from build123d import *

# Parameters (mm, degrees)
SKETCH1_R           = 46.5455
SKETCH1_R_2         = 2.60858
BOSS_EXTRUDE1_DEPTH = 3.1242
SKETCH1_5_R         = 47.498
SKETCH1_5_R_2       = 46.5455
BOSS_EXTRUDE2_DEPTH = 8.636
FILLET1_R           = 1.27
FILLET2_R           = 1.27
SKETCH2_R           = 46.4312
BOSS_EXTRUDE3_DEPTH = 0.508
SKETCH3_R           = 46.4312
BOSS_EXTRUDE4_DEPTH = 0.762


with BuildPart() as part:
    # Sketch1 → Boss-Extrude1 (new body)
    # profile 1 of 3: a face of its own
    with BuildSketch(Plane(origin=(0, 0, 0), x_dir=(1, 0, 0), z_dir=(0, 1, 0))):
        with Locations(Location((0, 0, 0), (0, 0, 270))):
            Circle(SKETCH1_R)
        Circle(SKETCH1_R_2, mode=Mode.SUBTRACT)
    # profile 2 of 3: a face of its own
    with BuildSketch(Plane(origin=(0, 0, 0), x_dir=(1, 0, 0), z_dir=(0, 1, 0))):
        with BuildLine():
            ThreePointArc((2.60858, 0), (2.193727268, 1.411470966), (1.081120394, 2.37399838))
            Line((1.081120394, 2.37399838), (2.175329976, -1.439662846))
            ThreePointArc((2.175329976, -1.439662846), (2.497920324, -0.751720475), (2.60858, 0))
        make_face()
    # profile 3 of 3: a face of its own
    with BuildSketch(Plane(origin=(0, 0, 0), x_dir=(1, 0, 0), z_dir=(0, 1, 0))):
        with BuildLine():
            Line((-1.081120394, -2.37399838), (-2.175329976, 1.439662846))
            ThreePointArc((-2.175329976, 1.439662846), (-2.507413058, -0.719422946), (-1.081120394, -2.37399838))
        make_face()
    extrude(amount=BOSS_EXTRUDE1_DEPTH)

    # Sketch1<5> → Boss-Extrude2 (add)
    with BuildSketch(Plane(origin=(0, 0, 0), x_dir=(1, 0, 0), z_dir=(0, 1, 0))):
        with Locations(Location((0, 0, 0), (0, 0, 270))):
            Circle(SKETCH1_5_R)
        with Locations(Location((0, 0, 0), (0, 0, 270))):
            Circle(SKETCH1_5_R_2, mode=Mode.SUBTRACT)
    extrude(amount=BOSS_EXTRUDE2_DEPTH)

    # Fillet1
    fillet1_edges = [part.edges().sort_by_distance(p)[0] for p in [
        (0, 0, -47.498),
    ]]
    fillet(fillet1_edges, radius=FILLET1_R)

    # Fillet2
    # the kernel refuses this fillet: 1.27 mm, written as the material it takes off along each edge
    with BuildSketch(Plane(origin=(0, 8.636, 0), x_dir=(0, 0, 1), z_dir=(-1, 0, 0))) as fillet2_piece_1:
        with BuildLine():
            CenterArc((46.228, -1.229672212), FILLET2_R, 0, 75.522487814)
            Line((46.5455, 0), (46.55185, 0.024593444))
            ThreePointArc((46.55185, 0.024593444), (47.02175, 0.0254), (47.498, 0.0254))
            Line((47.498, 0.0254), (47.5234, 0))
            Line((47.5234, 0), (47.5234, -1.229672212))
            Line((47.5234, -1.229672212), (47.498, -1.229672212))
        make_face()
    revolve(axis=Axis((0, 8.636, 0), (0, 1, 0)), mode=Mode.SUBTRACT)

    # Sketch2 → Boss-Extrude3 (add)
    with BuildSketch(Plane(origin=(0, 3.1242, 0), x_dir=(1, 0, 0), z_dir=(0, 1, 0))):
        with Locations(Location((0, 0, 0), (0, 0, 270))):
            Circle(SKETCH2_R)
        with BuildLine():
            Line((-1.081120394, -2.37399838), (-2.175329976, 1.439662846))
            ThreePointArc((-2.175329976, 1.439662846), (-0.719422946, 2.507413058), (1.081120394, 2.37399838))
            Line((1.081120394, 2.37399838), (2.175329976, -1.439662846))
            ThreePointArc((2.175329976, -1.439662846), (0.719422946, -2.507413058), (-1.081120394, -2.37399838))
        make_face(mode=Mode.SUBTRACT)
    extrude(amount=BOSS_EXTRUDE3_DEPTH)

    # Sketch3 → Boss-Extrude4 (add)
    with BuildSketch(Plane(origin=(0, 3.6322, 0), x_dir=(1, 0, 0), z_dir=(0, 1, 0))):
        with Locations(Location((0, 0, 0), (0, 0, 270))):
            Circle(SKETCH3_R)
    extrude(amount=BOSS_EXTRUDE4_DEPTH)


solid = part.part
Can you work these out from the model? Positions are in its coordinate system, mm. A direction names the side the tool comes from. Give positions to 0.01 mm unless a question says otherwise; leave off trailing zeros. Loops run counter-clockwise (first coordinate to the right, second up) from the corner with the lowest first, then second, coordinate; pieces in that order, holes last. Notation, with made-up numbers: (-30.75, 18) -> (-4.75, 18) arc R11 ccw to (-4.75, 33) -> close; hole circle Ø2 at (83, -7.5). An arc over 180 degrees is marked (long way). Write item = value, one per line.
1) Suppose I cut it at B-B on z = 0. Write out the boundary of the cut face in (x, y).
Check result:
outline = (-47.5, 1.27) arc R1.27 ccw to (-46.23, 0) -> (-1.76, 0) -> (-1.76, 3.63) -> (1.76, 3.63) -> (1.76, 0) -> (46.23, 0) arc R1.27 ccw to (47.5, 1.27) -> (47.5, 7.41) arc R1.27 ccw to (46.55, 8.64) -> (46.55, 3.12) -> (46.43, 3.12) -> (46.43, 4.39) -> (-46.43, 4.39) -> (-46.43, 3.12) -> (-46.55, 3.12) -> (-46.55, 8.64) arc R1.27 ccw to (-47.5, 7.41) -> close
2) Suppose I cut it at A-A on x = 0. Write out the boundary of the cut face in (y, z).
Check result:
outline = (0, -46.23) arc R1.27 ccw to (1.27, -47.5) -> (7.41, -47.5) arc R1.27 ccw to (8.64, -46.55) -> (3.12, -46.55) -> (3.12, -46.43) -> (4.39, -46.43) -> (4.39, 46.43) -> (3.12, 46.43) -> (3.12, 46.55) -> (8.64, 46.55) arc R1.27 ccw to (7.41, 47.5) -> (1.27, 47.5) arc R1.27 ccw to (0, 46.23) -> (0, 2.61) -> (3.63, 2.61) -> (3.63, -2.61) -> (0, -2.61) -> close
3) I need wall thicknesses on L1, parallel to X at y = 6.85, z = 0; L2, parallel to Y at x = 34, z = 31; L3, parallel to Z at x = -13.5, y = 5.25. Which ranges of each line are inside material? Lowest first, please. Write a range as from..to.
Check result:
L1 = -47.5..-46.55, 46.55..47.5
L2 = 0..4.39
L3 = -45.54..-44.54, 44.54..45.54
4) For faces 5 (the cylindrical face through (13.981, 5.842, 44.396)), 6 (the flat face through (-1.62, 1.79, 0.49)), which set-ups out of +Z, -Z, +X, -X, +Y, -Y let a thin tool reach every point of the face, with its end or its side?
Check result:
face_5 = +Y
face_6 = -Y
5) Thinking about a two-plate mould opening in Z: for faces 1 (the flat face through (1.62, 1.79, -0.49)), 2 (the flat face through (1, 4.394, -1)), 3 (the cylindrical face through (14.267, 4.295, 45.305)), 4 (the flat face through (1, 0, 10)), which applies, released by +Z, released by -Z, zero draft, split by the parting line, or undercut?
Check result:
face_1 = undercut
face_2 = undercut
face_3 = split by the parting line
face_4 = zero draft
6) Will these pins go through, and if not, where does the flat tip stop? pin 1 (12 mm diameter, centred on x = -31, z = 28, fed in from -Y); pin 2 (1.5 mm diameter, centred on x = -33.5, z = -4, fed in from +Y); pin 3 (2 mm diameter, centred on y = 7, z = 17.5, fed in from +X); pin 4 (5 mm diameter, centred on y = 3, z = -16.5, fed in from -X).
Check result:
pin_1 = 0
pin_2 = 4.39
pin_3 = 44.54
pin_4 = -45.39
